from build123d import *

# Parameters (mm, degrees)
ESQUISSE1_W                 = 45.287967496
ESQUISSE1_H                 = 7
BOSS_EXTRU_1_DEPTH          = 160
TROU_TARAUD_M41_D           = 3.3
TROU_TARAUD_M41_CSINK_D     = 4.05
TROU_TARAUD_M41_CSINK_ANGLE = 90
TROU_TARAUD_M53_D           = 4.2
TROU_TARAUD_M53_DEPTH       = 50
TROU_TARAUD_M53_CSINK_D     = 5.05
TROU_TARAUD_M53_CSINK_ANGLE = 90
TROU_TARAUD_M53_TIP         = 1.2618073


with BuildPart() as part:
    # Esquisse1 → Boss.-Extru.1 (new body)
    with BuildSketch(Plane.XY):
        with Locations((-5.5, -9.47)):
            Rectangle(ESQUISSE1_W, ESQUISSE1_H)
    extrude(amount=BOSS_EXTRU_1_DEPTH)

    # Trou taraudé M41 (through all)
    with Locations(Plane(origin=(0.354832292, -5.97, 0), x_dir=(1, 0, 0), z_dir=(0, 1, 0))):
        with Locations((-22.854832292, -20), (-22.854832292, -85), (-22.854832292, -150), (11.145167708, -150), (11.145167708, -85), (11.145167708, -20)):
            CounterSinkHole(TROU_TARAUD_M41_D / 2, TROU_TARAUD_M41_CSINK_D / 2, counter_sink_angle=TROU_TARAUD_M41_CSINK_ANGLE)

    # Trou taraudé M53
    with Locations(Plane(origin=(0, 0, 0), x_dir=(-1, 0, 0), z_dir=(0, 0, -1))):
        with Locations((5.5, -9.47)):
            CounterSinkHole(TROU_TARAUD_M53_D / 2, TROU_TARAUD_M53_CSINK_D / 2, depth=TROU_TARAUD_M53_DEPTH, counter_sink_angle=TROU_TARAUD_M53_CSINK_ANGLE)
            with Locations((0, 0, -(TROU_TARAUD_M53_DEPTH + TROU_TARAUD_M53_TIP / 2))):  # 118° drill point
                Cone(0, TROU_TARAUD_M53_D / 2, TROU_TARAUD_M53_TIP, mode=Mode.SUBTRACT)


solid = part.part
Can you work these out from the model? Positions are in its coordinate system, mm. A direction names the side the tool comes from. Round coordinates to 2 decimals unless told otherwise and drop trailing zeros. Order: outer loops, then holes, each group sorted by start corner. A loop starts at its lowest first (then second) coordinate and runs counter-clockwise, first axis right, second up. Notation, with made-up numbers: M 37,-19.75 L 53,-19.75 A14 cw 53,6.25 Z; hole C 31,77 d4. An arc over 180 degrees is marked long. Use a Markdown table: item, result.
1) If I drill on line 1 along Z through (x, y) = (11.5, -11); line 2 along X through (y, z) = (-10.5, 150); line 3 along X through (y, z) = (-9.25, 20), over which ranges is the centre line in solid material (lowest first)?
Geometry says:
| item | result |
|---|---|
| line 1 | z = 0 to 18.35, 21.65 to 83.35, 86.65 to 148.35, 151.65 to 160 |
| line 2 | x = -28.14 to -24.15, -20.85 to 9.85, 13.15 to 17.14 |
| line 3 | x = -28.14 to -24.15, -20.85 to -7.59, -3.41 to 9.85, 13.15 to 17.14 |
2) On a 3-axis mill with a long thin cutter (end or side, diameter ignored), from which of +Z, -Z, +X, -X, +Y, -Y can I reach the whole of each face in a straight line? I mean faces 4 (the face through (-5.96, -11.52, 25.56)), 5 (the face through (17.144, -10, 79)). Say none if no direction works.
Geometry says:
| item | result |
|---|---|
| face 4 | -Z |
| face 5 | +Z, -Z, +X, +Y, -Y |
3) Imagine slicing it at C-C (z = 85). List the corners of the cut face in (x, y) for me (3 decimals).
Geometry says:
| item | result |
|---|---|
| outline | M -28.144,-12.97 L -24.15,-12.97 L -24.15,-6.345 L -24.525,-5.97 L -28.144,-5.97 Z; M -20.85,-12.97 L 9.85,-12.97 L 9.85,-6.345 L 9.475,-5.97 L -20.475,-5.97 L -20.85,-6.345 Z; M 13.15,-12.97 L 17.144,-12.97 L 17.144,-5.97 L 13.525,-5.97 L 13.15,-6.345 Z |
4) If we mould it in two halves opening along Y, with no side actions, what happens to faces 1 (the face through (-5.453, -9.108, 51.043)), 2 (the face through (-21.19, -9.7, 86)), 3 (the face through (-6, -12.97, 79))? For each: +Y half, -Y half, draft (parallel to the pull), parting line (faces both ways), or undercut.
Geometry says:
| item | result |
|---|---|
| face 1 | undercut |
| face 2 | draft |
| face 3 | -Y half |
5) Imagine slicing it at B-B (x = 11.5). List the corners of the cut face in (y, z) for me (3 decimals), then the cut area to 3 significant figures.
Geometry says:
| item | result |
|---|---|
| outline | M -12.97,0 L -5.97,0 L -5.97,17.975 L -6.345,18.35 L -12.97,18.35 Z; M -12.97,21.65 L -6.345,21.65 L -5.97,22.025 L -5.97,82.975 L -6.345,83.35 L -12.97,83.35 Z; M -12.97,86.65 L -6.345,86.65 L -5.97,87.025 L -5.97,147.975 L -6.345,148.35 L -12.97,148.35 Z; M -12.97,151.65 L -6.345,151.65 L -5.97,152.025 L -5.97,160 L -12.97,160 Z |
| area | 1,050 mm² |
6) Imagine slicing it at A-A (z = 20). List the corners of the cut face in (x, y) for me (3 decimals).
Geometry says:
| item | result |
|---|---|
| outline | M -28.144,-12.97 L -24.15,-12.97 L -24.15,-6.345 L -24.525,-5.97 L -28.144,-5.97 Z; M -20.85,-12.97 L 9.85,-12.97 L 9.85,-6.345 L 9.475,-5.97 L -20.475,-5.97 L -20.85,-6.345 Z; M 13.15,-12.97 L 17.144,-12.97 L 17.144,-5.97 L 13.525,-5.97 L 13.15,-6.345 Z; hole C -5.5,-9.47 d4.2 |
